Can you work these out from the model? Positions are in its coordinate system, mm. A direction names the side the tool comes from. Coordinates: 2 decimals unless noted, no trailing zeros. Order: outer loops, then holes, each group sorted by start corner. A loop starts at its lowest first (then second) coordinate and runs counter-clockwise, first axis right, second up. Notation, with made-up numbers: (65, -8.75) - (86, -8.75) arc R15 ccw to (86, 11.25) - close; hole circle Ø7 at (36, -37.5). An arc over 180 degrees is marked (long way). Return JSON: item names as keys, results as strings. Group by question number.
1) If I drill on line 1 along Y through (x, z) = (2.5, 8); line 2 along X through (y, z) = (0.5, 7.25); line 3 along Y through (x, z) = (28.5, 2.25), over which ranges is the centre line in solid material (lowest first)?
2) Which directions (+Z, -Z, +X, -X, +Y, -Y) give clear straight access to the entire face, cutting with the end or side of a thin tool? Please do faces 1 (the face through (-31, -14, 8)), 2 (the face through (0, -15.5, 8)).
3) Imagine slicing it at A-A (y = 4). Write out the boundary of the cut face in (x, z).
4) Imagine slicing it at B-B (x = -5.5). Write out the boundary of the cut face in (y, z), and give its area (3 significant figures).
5) For pin 1 Ø6 at (x, y) = (-16, 4) entering from +Z, with a flat end and sliding along its axis, tell me the tip position at first contact or that it passes through.
6) If we mould it in two halves opening along X, with no side actions, what happens to faces 3 (the face through (0.48, -15.07, 0.45)), 4 (the face through (-28, 12.5, 8))? For each: pulls with the +X half, pulls with the -X half, needs draft (parallel to the pull), parting line crosses it, or undercut.
Autodesk Inventor part; units mm, degrees
ref_plane "YZ Plane" through (0, 0, 0) normal (1, 0, 0) x (0, 1, 0)
ref_plane "XZ Plane" through (0, 0, 0) normal (0, 1, 0) x (-1, 0, 0)
ref_plane "XY Plane" through (0, 0, 0) normal (0, 0, 1) x (1, 0, 0)
sketch "Skizze2" plane through (0, 0, 0) normal (0, 0, 1) x (1, 0, 0)
  line L0 (-32.5, 14) -> (32.5, 14)
  line L1 (32.5, 14) -> (32.5, -14)
  line L2 (32.5, -14) -> (-32.5, -14)
  line L3 (-32.5, -14) -> (-32.5, 14)
  line L4 (-32.5, 14) -> (32.5, -14) construction
  line L5 (32.5, 14) -> (-32.5, -14) construction
  point P0 (0, 0)
  dimension "d0" = 65
  dimension "d1" = 28
extrude "Extrusion1" add sketch "Skizze2" along normal blind 1.5
sketch "Skizze4" plane through (0, 0, 0) normal (0, 0, -1) x (-1, 0, 0)
  line L0 (32.5, 14) -> (-32.5, 14)
  line L1 (-32.5, 14) -> (-32.5, -14)
  line L2 (-32.5, -14) -> (32.5, -14)
  line L3 (32.5, -14) -> (32.5, 14)
  line L4 (34, -15.5) -> (-34, -15.5)
  line L5 (-34, -15.5) -> (-34, 15.5)
  line L6 (-34, 15.5) -> (34, 15.5)
  line L7 (34, 15.5) -> (34, -15.5)
  point P0 (0, 0)
  dimension "d4" = 1.5
extrude "Extrusion2" add sketch "Skizze4" against normal blind 14
fillet "Rundung1" radius 1.5 4 edges at (0, -15.5, 0) (0, 15.5, 0) (34, 0, 0) (-34, 0, 0)
sketch "Skizze5" plane through (0, 0, 1.5) normal (0, 0, 1) x (1, 0, 0)
  line L0 (0, -21.0221) -> (0, 21.9802) construction
  line L1 (-32.5, -14) -> (32.5, -14)
  line L2 (-28.7599, -14) -> (-26.7599, -14)
  line L3 (-26.7599, -14) -> (-26.7599, -12.5)
  line L4 (-26.7599, -12.5) -> (-28.7599, -12.5)
  line L5 (-28.7599, -12.5) -> (-28.7599, -14)
  line L6 (-24.7599, -14) -> (-22.7599, -14)
  line L7 (-22.7599, -14) -> (-22.7599, -12.5)
  line L8 (-22.7599, -12.5) -> (-24.7599, -12.5)
  line L9 (-24.7599, -12.5) -> (-24.7599, -14)
  line L10 (-34, 15.5) -> (-34, -15.5) construction
  line L11 (-34, 0) -> (34, 0) construction
  line L12 (34, -15.5) -> (34, 15.5) construction
  line L13 (28.7599, -14) -> (26.7599, -14)
  line L14 (26.7599, -14) -> (26.7599, -12.5)
  line L15 (26.7599, -12.5) -> (28.7599, -12.5)
  line L16 (28.7599, -12.5) -> (28.7599, -14)
  line L17 (24.7599, -14) -> (22.7599, -14)
  line L18 (22.7599, -14) -> (22.7599, -12.5)
  line L19 (22.7599, -12.5) -> (24.7599, -12.5)
  line L20 (24.7599, -12.5) -> (24.7599, -14)
  line L21 (34, 15.5) -> (34, -15.5) construction
  line L22 (-28.7599, 14) -> (-26.7599, 14)
  line L23 (-26.7599, 14) -> (-26.7599, 12.5)
  line L24 (-26.7599, 12.5) -> (-28.7599, 12.5)
  line L25 (-28.7599, 12.5) -> (-28.7599, 14)
  line L26 (-24.7599, 14) -> (-22.7599, 14)
  line L27 (-22.7599, 14) -> (-22.7599, 12.5)
  line L28 (-22.7599, 12.5) -> (-24.7599, 12.5)
  line L29 (-24.7599, 12.5) -> (-24.7599, 14)
  line L30 (22.7599, 14) -> (22.7599, 12.5)
  line L31 (24.7599, 14) -> (22.7599, 14)
  line L32 (22.7599, 12.5) -> (24.7599, 12.5)
  line L33 (24.7599, 12.5) -> (24.7599, 14)
  line L34 (26.7599, 14) -> (26.7599, 12.5)
  line L35 (28.7599, 14) -> (26.7599, 14)
  line L36 (26.7599, 12.5) -> (28.7599, 12.5)
  line L37 (28.7599, 12.5) -> (28.7599, 14)
  point P0 (0, 0)
  dimension "d11" = 2
  dimension "d12" = 1.5
  dimension "d13" = 2
  dimension "d14" = 2
extrude "Extrusion4" add sketch "Skizze5" along normal blind 12.5
properties part number "Unterteil"
Calculated:
{
 "1": {"line 1": "-15.5 to -14, 14 to 15.5", "line 2": "-34 to -32.5, 32.5 to 34", "line 3": "-15.5 to -12.5, 12.5 to 15.5"},
 "2": {"face 1": "+Z", "face 2": "+Z, -Z, +X, -X, -Y"},
 "3": {"outline": "(-34, 1.5) arc R1.5 ccw to (-32.5, 0) - (32.5, 0) arc R1.5 ccw to (34, 1.5) - (34, 14) - (32.5, 14) - (32.5, 1.5) - (-32.5, 1.5) - (-32.5, 14) - (-34, 14) - close"},
 "4": {"outline": "(-15.5, 1.5) arc R1.5 ccw to (-14, 0) - (14, 0) arc R1.5 ccw to (15.5, 1.5) - (15.5, 14) - (14, 14) - (14, 1.5) - (-14, 1.5) - (-14, 14) - (-15.5, 14) - close", "area": "83.0 mm2"},
 "5": {"pin 1": "z = 1.5"},
 "6": {"face 3": "needs draft", "face 4": "undercut"}
}
